```python
from build123d import *

# Parameters (mm, degrees)
EXTRUDE_1_DEPTH     = 4
SKETCH_2_W          = 1.5
SKETCH_2_H          = 40.43
EXTRUDE_2_DEPTH     = 1.5
SKETCH_3_W          = 40.43
SKETCH_3_H          = 1.5
EXTRUDE_5_DEPTH     = 54.71
SKETCH_4_W          = 40.43
SKETCH_4_H          = 1.5
CUT_EXTRUDE_1_DEPTH = 20.3
SKETCH_5_W          = 6.5
SKETCH_5_H          = 1.5
EXTRUDE_6_DEPTH     = 20.3
SKETCH_6_R          = 0.8
CUT_EXTRUDE_2_DEPTH = 20.3
SKETCH_7_R          = 2.333452378
CUT_EXTRUDE_5_DEPTH = 1
CUT_EXTRUDE_6_DEPTH = 10


with BuildPart() as part:
    # 草图1 → 凸台-拉伸1 (new body)
    with BuildSketch(Plane(origin=(0, 0, 0), x_dir=(1, 0, 0), z_dir=(0, 1, 0))):
        Polygon((-13.121987947, 19.52916985), (-7.621987947, 19.52916985), (-7.621987947, 22.82916985), (-63.831987947, 22.82916985), (-63.831987947, -17.60083015), (-7.621987947, -17.60083015), (-7.621987947, -14.30083015), (-13.121987947, -14.30083015), (-13.121987947, -16.10083015), (-60.331987947, -16.10083015), (-60.331987947, -14.30083015), (-62.331987947, -14.30083015), (-62.331987947, 19.52916985), (-60.331987947, 19.52916985), (-60.331987947, 21.32916985), (-13.121987947, 21.32916985), align=None)
    extrude(amount=EXTRUDE_1_DEPTH)

    # 草图2 → 凸台-拉伸2 (add)
    with BuildSketch(Plane(origin=(0, 4, 0), x_dir=(1, 0, 0), z_dir=(0, 1, 0))):
        with Locations((-63.081987947, 2.61416985)):
            Rectangle(SKETCH_2_W, SKETCH_2_H)
    extrude(amount=EXTRUDE_2_DEPTH)

    # 草图3 → 凸台-拉伸5 (add)
    with BuildSketch(Plane(origin=(-62.331987947, 0, 0), x_dir=(0, 0, -1), z_dir=(1, 0, 0))):
        with Locations((2.61416985, 4.75)):
            Rectangle(SKETCH_3_W, SKETCH_3_H)
    extrude(amount=EXTRUDE_5_DEPTH)

    # 草图4 → 切除-拉伸1 (cut)
    with BuildSketch(Plane(origin=(-7.621987947, 0, 0), x_dir=(0, 0, -1), z_dir=(1, 0, 0))):
        with Locations((2.61416985, 4.75)):
            Rectangle(SKETCH_4_W, SKETCH_4_H)
    extrude(amount=-CUT_EXTRUDE_1_DEPTH, mode=Mode.SUBTRACT)

    # 草图5 → 凸台-拉伸6 (add)
    with BuildSketch(Plane(origin=(-27.921987947, 0, 0), x_dir=(0, 0, -1), z_dir=(1, 0, 0))):
        with Locations((-14.35083015, 4.75)):
            Rectangle(SKETCH_5_W, SKETCH_5_H)
        with Locations((19.57916985, 4.75)):
            Rectangle(SKETCH_5_W, SKETCH_5_H)
    extrude(amount=EXTRUDE_6_DEPTH)

    # 草图6 → 切除-拉伸2 (cut)
    with BuildSketch(Plane.XZ):
        with Locations(Location((-9.271987947, -21.17916985, 0), (0, 0, 270))):
            Circle(SKETCH_6_R)
        with Locations(Location((-9.271987947, 15.95083015, 0), (0, 0, 270))):
            Circle(SKETCH_6_R)
        with Locations(Location((-62.181987947, 15.95083015, 0), (0, 0, 270))):
            Circle(SKETCH_6_R)
        with Locations(Location((-62.181987947, -21.17916985, 0), (0, 0, 270))):
            Circle(SKETCH_6_R)
    extrude(amount=-CUT_EXTRUDE_2_DEPTH, mode=Mode.SUBTRACT)

    # 草图7 → 切除-拉伸5 (cut)
    with BuildSketch(Plane(origin=(0, 5.5, 0), x_dir=(1, 0, 0), z_dir=(0, 1, 0))):
        with Locations((-62.181987947, -15.95083015)):
            Circle(SKETCH_7_R)
        with Locations((-62.181987947, 21.17916985)):
            Circle(SKETCH_7_R)
        with Locations((-9.271987947, 21.17916985)):
            Circle(SKETCH_7_R)
        with Locations((-9.271987947, -15.95083015)):
            Circle(SKETCH_7_R)
    extrude(amount=-CUT_EXTRUDE_5_DEPTH, mode=Mode.SUBTRACT)

    # 草图9 → 切除-拉伸6 (cut)
    with BuildSketch(Plane.XZ):
        with BuildLine():
            Line((-62.747673372, -22.82916985), (-63.831987947, -22.82916985))
            Line((-63.831987947, -22.82916985), (-63.831987947, -21.744855275))
            ThreePointArc((-63.831987947, -21.744855275), (-63.514399561, -22.511581464), (-62.747673372, -22.82916985))
        make_face()
        with BuildLine():
            Line((-62.747673372, 17.60083015), (-63.831987947, 17.60083015))
            Line((-63.831987947, 17.60083015), (-63.831987947, 16.516515575))
            ThreePointArc((-63.831987947, 16.516515575), (-63.514399561, 17.283241764), (-62.747673372, 17.60083015))
        make_face()
        with BuildLine():
            Line((-7.621987947, 16.516515575), (-7.621987947, 17.60083015))
            Line((-7.621987947, 17.60083015), (-8.706302522, 17.60083015))
            ThreePointArc((-8.706302522, 17.60083015), (-7.939576333, 17.283241764), (-7.621987947, 16.516515575))
        make_face()
        with BuildLine():
            Line((-7.621987947, -21.744855275), (-7.621987947, -22.82916985))
            Line((-7.621987947, -22.82916985), (-8.706302522, -22.82916985))
            ThreePointArc((-8.706302522, -22.82916985), (-7.939576333, -22.511581464), (-7.621987947, -21.744855275))
        make_face()
    extrude(amount=-CUT_EXTRUDE_6_DEPTH, mode=Mode.SUBTRACT)


solid = part.part
```
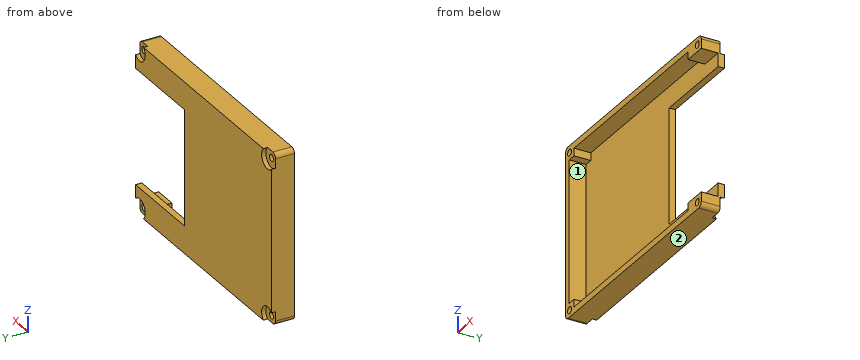
Build history of the part. All positions in model axes, mm. Face numbers are marked on the shaded views. A direction names the side the tool comes from. Round coordinates to 2 decimals unless told otherwise and drop trailing zeros. Order: outer loops, then holes, each group sorted by start corner. A loop starts at its lowest first (then second) coordinate and runs counter-clockwise, first axis right, second up. Notation, with made-up numbers: (48, -1.5) - (79, -1.5) arc R18 cw to (79, 16.5) - close; hole circle Ø7 at (43.25, 44.25). An arc over 180 degrees is marked (long way). Use a Markdown table: item, result.
1) Saw through at A-A on x = -24.5. Write the cut outline in (y, z).
Recorded:
| item | result |
|---|---|
| outline | (0, -22.83) - (5.5, -22.83) - (5.5, -16.33) - (4, -16.33) - (4, -21.33) - (0, -21.33) - close; (0, 16.1) - (4, 16.1) - (4, 11.1) - (5.5, 11.1) - (5.5, 17.6) - (0, 17.6) - close |
2) Tool access for the marked faces 1 and 2: list every direction of +Z, -Z, +X, -X, +Y, -Y with a clear straight run to the whole face (end or side of a thin tool).
Recorded:
| item | result |
|---|---|
| face 1 | +X, -Y |
| face 2 | -Z, +X, -X, +Y, -Y |
3) Wall check: L1, parallel to X at y = 0.7, z = 16; L2, parallel to Z at x = -12, y = 2.25; L3, parallel to Z at x = -49.5, y = 1. Give the ranges that are in metal, low to high.
Recorded:
| item | result |
|---|---|
| L1 | x = -63.83 to -62.98, -61.38 to -60.33, -13.12 to -10.07, -8.47 to -7.62 |
| L2 | z = -22.83 to -19.53, 14.3 to 17.6 |
| L3 | z = -22.83 to -21.33, 16.1 to 17.6 |
4) Saw through at B-B on x = -52.5. Write the cut outline in (y, z).
Recorded:
| item | result |
|---|---|
| outline | (0, -22.83) - (5.5, -22.83) - (5.5, 17.6) - (0, 17.6) - (0, 16.1) - (4, 16.1) - (4, -21.33) - (0, -21.33) - close |
5) Saw through at D-D on y = 3.3. Write the cut outline in (x, z).
Recorded:
| item | result |
|---|---|
| outline | (-63.83, -21.74) arc R1.08 ccw to (-62.75, -22.83) - (-8.71, -22.83) arc R1.08 ccw to (-7.62, -21.74) - (-7.62, -19.53) - (-13.12, -19.53) - (-13.12, -21.33) - (-60.33, -21.33) - (-60.33, -19.53) - (-62.33, -19.53) - (-62.33, 14.3) - (-60.33, 14.3) - (-60.33, 16.1) - (-13.12, 16.1) - (-13.12, 14.3) - (-7.62, 14.3) - (-7.62, 16.52) arc R1.08 ccw to (-8.71, 17.6) - (-62.75, 17.6) arc R1.08 ccw to (-63.83, 16.52) - close; hole circle Ø1.6 at (-62.18, -21.18); hole circle Ø1.6 at (-62.18, 15.95); hole circle Ø1.6 at (-9.27, -21.18); hole circle Ø1.6 at (-9.27, 15.95) |
6) Saw through at C-C on z = 9. Write the cut outline in (x, y), and give its area (3 significant figures).
Recorded:
| item | result |
|---|---|
| outline | (-63.83, 0) - (-62.33, 0) - (-62.33, 4) - (-27.92, 4) - (-27.92, 5.5) - (-63.83, 5.5) - close |
| area | 59.9 mm² |
7) Flat gauge pins, fed straight in: pin 1 Ø1.5 at (x, z) = (-18.5, 10) entering from +Y; pin 2 Ø0.8 at (y, z) = (5, 3) entering from +X; pin 3 Ø2 at (x, z) = (-28, -10) entering from -Y; pin 4 Ø2 at (x, z) = (-9, -20) entering from +Y. Where does each tip first touch, or does it go through?
Recorded:
| item | result |
|---|---|
| pin 1 | passes through |
| pin 2 | stops at x = -27.92 |
| pin 3 | stops at y = 4 |
| pin 4 | stops at y = 4.5 |
